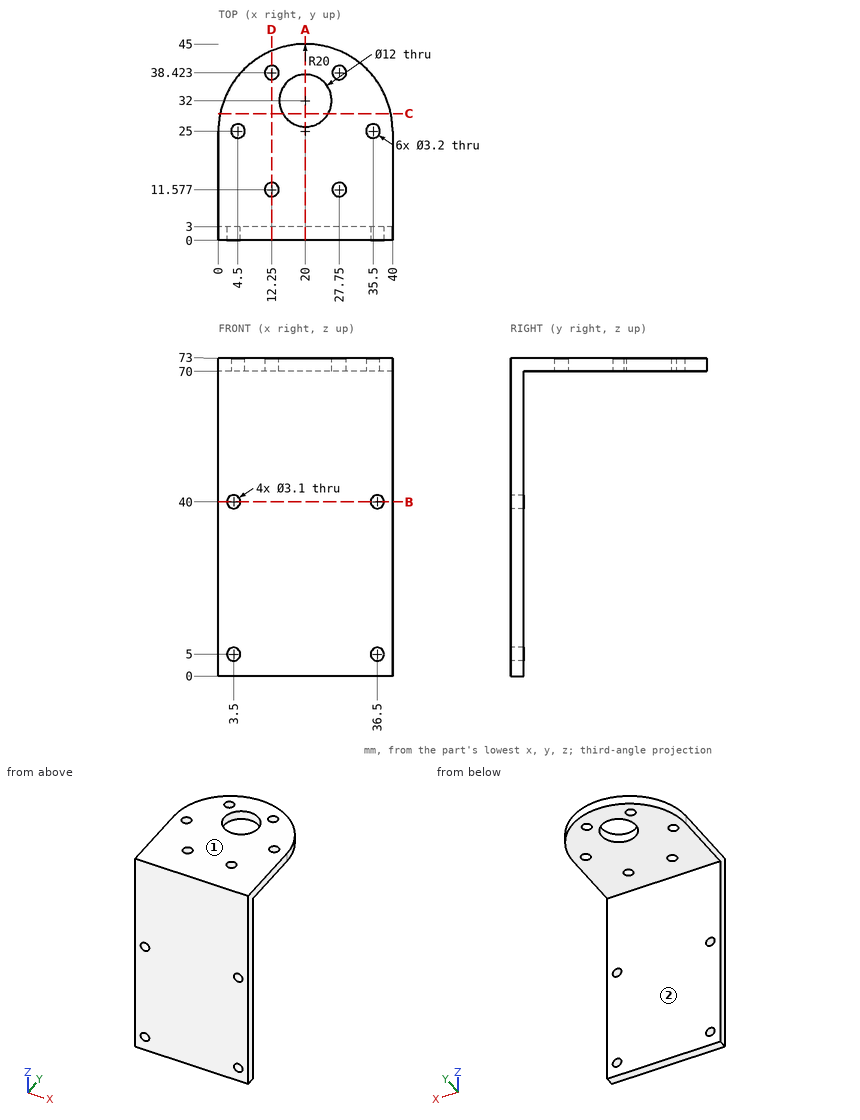
Geometry check sheet. Reference: drawing and pictorial views, mm from the part's lowest x, y, z. A direction names the side the tool comes from. Give positions to 0.01 mm unless a question says otherwise; leave off trailing zeros. Order: outer loops, then holes, each group sorted by start corner. A loop starts at its lowest first (then second) coordinate and runs counter-clockwise, first axis right, second up. Notation, with made-up numbers: M 89,59.5 L 122,59.5 A16 cw 122,74.5 Z; hole C -23,52 d9. An arc over 180 degrees is marked long. Answer in a Markdown table with one row per item. Add a question column.
Q1. Gauge pin test, flat ends, axial feed: pin 1 Ø8 at (x, y) = (20, 12) entering from -Z; pin 2 Ø12 at (x, z) = (11.5, 44.5) entering from +Y; pin 3 Ø2.5 at (x, y) = (12.25, 38.42) entering from -Z. Record the tip position at first contact, or that the pin passes through.
Q2. Sectioned sample at A-A, the plane x = 20. Record the boundary of the cut face in (y, z).
Q3. Sectioned sample at D-D, the plane x = 12.25. Record the boundary of the cut face in (y, z).
Q4. Sectioned sample at C-C, the plane y = 29. Record the boundary of the cut face in (x, z).
Q5. Thickness scan on L1, parallel to Z at x = 36.5, y = 1.8; L2, parallel to Y at x = 27.75, z = 72.2; L3, parallel to Y at x = 20, z = 71. Record the ranges inside material, lowest first.
Q6. Sectioned sample at B-B, the plane z = 40. Record the boundary of the cut face in (x, y).
Q7. Access from +Z, -Z, +X, -X, +Y, -Y to the whole of each face (thin tool, end or side, straight path). Record for the marked faces 1 and 2.
Verdict:
| question | item | result |
|---|---|---|
| 1 | pin 1 | z = 70 |
| 1 | pin 2 | y = 3 |
| 1 | pin 3 | through |
| 2 | outline | M 0,0 L 3,0 L 3,70 L 26,70 L 26,73 L 0,73 Z; M 38,70 L 45,70 L 45,73 L 38,73 Z |
| 3 | outline | M 0,0 L 3,0 L 3,70 L 9.98,70 L 9.98,73 L 0,73 Z; M 13.18,70 L 36.82,70 L 36.82,73 L 13.18,73 Z; M 40.02,70 L 43.44,70 L 43.44,73 L 40.02,73 Z |
| 4 | outline | M 0.4,70 L 14.8,70 L 14.8,73 L 0.4,73 Z; M 25.2,70 L 39.6,70 L 39.6,73 L 25.2,73 Z |
| 5 | L1 | 0 to 3.45, 6.55 to 38.45, 41.55 to 73 |
| 5 | L2 | 0 to 9.98, 13.18 to 36.82, 40.02 to 43.44 |
| 5 | L3 | 0 to 26, 38 to 45 |
| 6 | outline | M 0,0 L 1.95,0 L 1.95,3 L 0,3 Z; M 5.05,0 L 34.95,0 L 34.95,3 L 5.05,3 Z; M 38.05,0 L 40,0 L 40,3 L 38.05,3 Z |
| 7 | face 1 | +Z, +X, -X, +Y, -Y |
| 7 | face 2 | -Z, +X, -X, +Y |
